from build123d import *

# Parameters (mm, degrees)
SKETCH1_R           = 5
BOSS_EXTRUDE1_DEPTH = 10
SKETCH3_R           = 2.5
SKETCH3_W           = 43
SKETCH3_H           = 28
CUT_EXTRUDE1_DEPTH  = 126.574678976
FILLET1_R           = 10
FILLET2_R           = 10
BOSS_EXTRUDE2_DEPTH = 87
SKETCH4_4_R         = 12.5
CUT_EXTRUDE3_DEPTH  = 87
FILLET3_R           = 10
SKETCH8_W           = 40
SKETCH8_H           = 23.261660468
CUT_EXTRUDE8_DEPTH  = 87
SKETCH9_W           = 20
SKETCH9_H           = 10
BOSS_EXTRUDE3_DEPTH = 87
FILLET4_R           = 5
SKETCH10_R          = 3.175
CUT_EXTRUDE9_DEPTH  = 126.574678976
FILLET5_R           = 5
SKETCH11_R          = 7
CUT_EXTRUDE10_DEPTH = 126.574678976


with BuildPart() as part:
    # Sketch1 → Boss-Extrude1 (new body)
    with BuildSketch(Plane(origin=(0, 0, 0), x_dir=(1, 0, 0), z_dir=(0, 1, 0))):
        Polygon((0, 90), (15.718723237, 90), (15.718723237, 74), (70.870392539, 74), (70.870392539, 90), (87, 90), (87, 0), (0, 0), align=None)
        with Locations(Location((10, 74, 0), (0, 0, 270))):
            Circle(SKETCH1_R, mode=Mode.SUBTRACT)
        with Locations(Location((77, 74, 0), (0, 0, 270))):
            Circle(SKETCH1_R, mode=Mode.SUBTRACT)
    extrude(amount=BOSS_EXTRUDE1_DEPTH)

    # Sketch3 → Cut-Extrude1 (cut, through all)
    with BuildSketch(Plane(origin=(0, 10, 0), x_dir=(1, 0, 0), z_dir=(0, 1, 0))):
        with Locations(Location((19.6, 53, 0), (0, 0, 270))):
            Circle(SKETCH3_R)
        with Locations(Location((70.4, 62.836666102, 0), (0, 0, 270))):
            Circle(SKETCH3_R)
        with Locations(Location((70.4, 52.836666102, 0), (0, 0, 270))):
            Circle(SKETCH3_R)
        with Locations((44.9, 60)):
            Rectangle(SKETCH3_W, SKETCH3_H)
        with Locations(Location((19.6, 62.836666102, 0), (0, 0, 270))):
            Circle(SKETCH3_R)
    extrude(amount=-CUT_EXTRUDE1_DEPTH, mode=Mode.SUBTRACT)

    # Fillet1
    # the kernel refuses this fillet: 10 mm, written as the material it adds along each edge
    with BuildSketch(Plane(origin=(70.870392539, 0, -74), x_dir=(0, 0, -1), z_dir=(0, 1, 0))) as fillet1_piece_1:
        with BuildLine():
            CenterArc((8.332073051, 10), FILLET1_R, 213.570370594, 56.429629406)
            Line((0, 4.470392539), (-0.166641461, 4.359800389))
            ThreePointArc((-0.166641461, 4.359800389), (-0.2, 2.235196269), (-0.2, 0))
            Line((-0.2, 0), (0, -0.2))
            Line((0, -0.2), (8.332073051, -0.2))
            Line((8.332073051, -0.2), (8.332073051, 0))
        make_face()
    extrude(amount=10)
    with BuildSketch(Plane(origin=(15.718723237, 0, -74), x_dir=(0, 0, -1), z_dir=(0, 1, 0))) as fillet1_piece_2:
        with BuildLine():
            CenterArc((9.727462287, -10), FILLET1_R, 90, 76.592671632)
            Line((0, -7.681276763), (-0.194549246, -7.634902298))
            ThreePointArc((-0.194549246, -7.634902298), (-0.2, -3.840638382), (-0.2, 0))
            Line((-0.2, 0), (0, 0.2))
            Line((0, 0.2), (9.727462287, 0.2))
            Line((9.727462287, 0.2), (9.727462287, 0))
        make_face()
    extrude(amount=10)

    # Fillet2
    fillet2_edges = [part.edges().sort_by_distance(p)[0] for p in [
        (66.4, 5, -74),
        (23.4, 5, -74),
    ]]
    fillet(fillet2_edges, radius=FILLET2_R)

    # Sketch4 → Boss-Extrude2 (add)
    with BuildSketch(Plane(origin=(87, 0, 0), x_dir=(0, 0, -1), z_dir=(1, 0, 0))):
        with BuildLine():
            Line((36, 0), (0, 0))
            Line((0, 0), (0, 10))
            Line((0, 10), (8.5, 10))
            ThreePointArc((8.5, 10), (16, 12.5), (23.5, 10))
            Line((23.5, 10), (33.320508076, 10))
            ThreePointArc((33.320508076, 10), (-3.318516526, -5.176380902), (36, 0))
        make_face()
    extrude(amount=-BOSS_EXTRUDE2_DEPTH)

    # Sketch4<4> → Cut-Extrude3 (cut)
    with BuildSketch(Plane(origin=(87, 0, 0), x_dir=(0, 0, -1), z_dir=(1, 0, 0))):
        with Locations((16, 0)):
            Circle(SKETCH4_4_R)
    extrude(amount=-CUT_EXTRUDE3_DEPTH, mode=Mode.SUBTRACT)

    # Fillet3
    fillet3_edges = [part.edges().sort_by_distance(p)[0] for p in [
        (43.5, 10, -33.320508076),
    ]]
    fillet(fillet3_edges, radius=FILLET3_R)

    # Sketch8 → Cut-Extrude8 (cut)
    with BuildSketch(Plane(origin=(87, 0, 0), x_dir=(0, 0, -1), z_dir=(1, 0, 0))):
        with Locations((16, -11.630830234)):
            Rectangle(SKETCH8_W, SKETCH8_H)
    extrude(amount=-CUT_EXTRUDE8_DEPTH, mode=Mode.SUBTRACT)

    # Sketch9 → Boss-Extrude3 (add)
    with BuildSketch(Plane(origin=(87, 0, 0), x_dir=(0, 0, -1), z_dir=(1, 0, 0))):
        with Locations((-6.5, 5)):
            Rectangle(SKETCH9_W, SKETCH9_H)
    extrude(amount=-BOSS_EXTRUDE3_DEPTH)

    # Fillet4
    fillet4_edges = [part.edges().sort_by_distance(p)[0] for p in [
        (43.5, 10, 16.5),
    ]]
    fillet(fillet4_edges, radius=FILLET4_R)

    # Sketch10 → Cut-Extrude9 (cut, through all)
    with BuildSketch(Plane(origin=(0, 10, 0), x_dir=(1, 0, 0), z_dir=(0, 1, 0))):
        with Locations(Location((15.718723237, -6.5, 0), (0, 0, 270))):
            Circle(SKETCH10_R)
        with Locations(Location((70.870392539, -6.5, 0), (0, 0, 270))):
            Circle(SKETCH10_R)
    extrude(amount=-CUT_EXTRUDE9_DEPTH, mode=Mode.SUBTRACT)

    # Fillet5
    fillet5_edges = [part.edges().sort_by_distance(p)[0] for p in [
        (0, 5, -90),
        (87, 5, -90),
    ]]
    fillet(fillet5_edges, radius=FILLET5_R)

    # Sketch11 → Cut-Extrude10 (cut, through all)
    with BuildSketch(Plane(origin=(0, 10, 0), x_dir=(1, 0, 0), z_dir=(0, 1, 0))):
        with Locations((15.718723237, -6.5)):
            Circle(SKETCH11_R)
        with Locations((70.870392539, -6.5)):
            Circle(SKETCH11_R)
    extrude(amount=CUT_EXTRUDE10_DEPTH, mode=Mode.SUBTRACT)


solid = part.part
Model file for the job. Use its own axes, mm. A direction names the side the tool comes from. Round coordinates to 2 decimals unless told otherwise and drop trailing zeros. Order: outer loops, then holes, each group sorted by start corner. A loop starts at its lowest first (then second) coordinate and runs counter-clockwise, first axis right, second up. Notation, with made-up numbers: M 45,49.5 L 58,49.5 A4 cw 58,53.5 Z; hole C 29,55.5 d4. An arc over 180 degrees is marked long. Write each question's results on one line, items separated by ' | '. Start each with the question number.
(1) Drop flat-ended pins along their axis: pin 1 (12 mm diameter, centred on x = 49.5, y = 7, fed in from -Z); pin 2 (6.5 mm diameter, centred on x = 70.4, z = -62.84, fed in from +Y); pin 3 (5 mm diameter, centred on x = 39.5, y = 10, fed in from +Z); pin 4 (5.5 mm diameter, centred on x = 70.87, z = 6.5, fed in from +Y). Give the stop position or say it passes through.
(2) Saw through at B-B, the plane y = 1.5. State how many separate pieces and enclosed holes the cut face has, then the cut area to 3 significant figures.
(3) Which spindle directions (+Z, -Z, +X, -X, +Y, -Y) get a long thin tool onto all of the face, cutting with end or side? Do faces 4 (the face through (23.4, 5, -57)), 5 (the face through (68.182, 5.07, -51.683)), 6 (the face through (15.8, 11, -0.5)). Say none if no direction does.
(4) Saw through at C-C, the plane x = 32. Give the cut face in (y, z), then the cut area to 3 significant figures.
(5) Two-plate mould, pull along Z, no slides. Class faces 1 (the face through (18.64, 5.07, -50.69)), 2 (the face through (44, 2, 16.5)), 3 (the face through (1, 5, -88)): pulls with the +Z half, pulls with the -Z half, needs draft (parallel to the pull), parting line crosses it, or undercut.
(6) Saw through at D-D, the plane z = -72. Give the cut face in (x, y), then the cut area to 3 significant figures.
(7) Saw through at A-A, the plane z = 6.5. Give the cut face in (x, y), then the cut area to 3 significant figures.
(8) Probe probe 1 along X at (y, z) = (4, -66.5); probe 2 along Y at (x, z) = (82.5, -62.5); probe 3 along Z at (x, y) = (49, 1). List the from-to ranges inside material, lowest first. Write a range as from..to.
Established:
1) pin 1: stops at z = -46 | pin 2: stops at y = 10 | pin 3: stops at z = 15.83 | pin 4: passes through
2) separate pieces: 2 | enclosed holes: 8 | area: 4,730 mm^2
3) face 4: -Z, +Y, -Y | face 5: +Y, -Y | face 6: +Z, +Y
4) outline: M 0,-46 L 10,-46 L 10,-38.36 A10 cw 13.33,-30.91 A20 ccw 10,1.32 L 10,11.5 A5 ccw 5,16.5 L 0,16.5 L 0,-3.5 A12.5 cw 0,-28.5 Z | area: 623 mm^2
5) face 1: undercut | face 2: pulls with the +Z half | face 3: pulls with the -Z half
6) outline: M 0,0 L 5.42,0 L 5.42,10 L 0,10 Z; M 14.58,0 L 22.55,0 L 22.55,10 L 14.58,10 Z; M 66.66,0 L 72.42,0 L 72.42,10 L 66.66,10 Z; M 81.58,0 L 87,0 L 87,10 L 81.58,10 Z | area: 246 mm^2
7) outline: M 0,0 L 12.54,0 L 12.54,10 L 0,10 Z; M 18.89,0 L 67.7,0 L 67.7,10 L 18.89,10 Z; M 74.05,0 L 87,0 L 87,10 L 74.05,10 Z | area: 743 mm^2
8) probe 1: x = 0..23.4, 66.4..87 | probe 2: y = 0..10 | probe 3: z = -46..-28.46, -3.54..16.5
